Could you check a few things on this drawing? It's one solid part, dimensions in mm from its lowest x, y, z. A direction names the side the tool comes from. Give positions to 0.01 mm unless a question says otherwise; leave off trailing zeros. Order: outer loops, then holes, each group sorted by start corner. A loop starts at its lowest first (then second) coordinate and runs counter-clockwise, first axis right, second up.
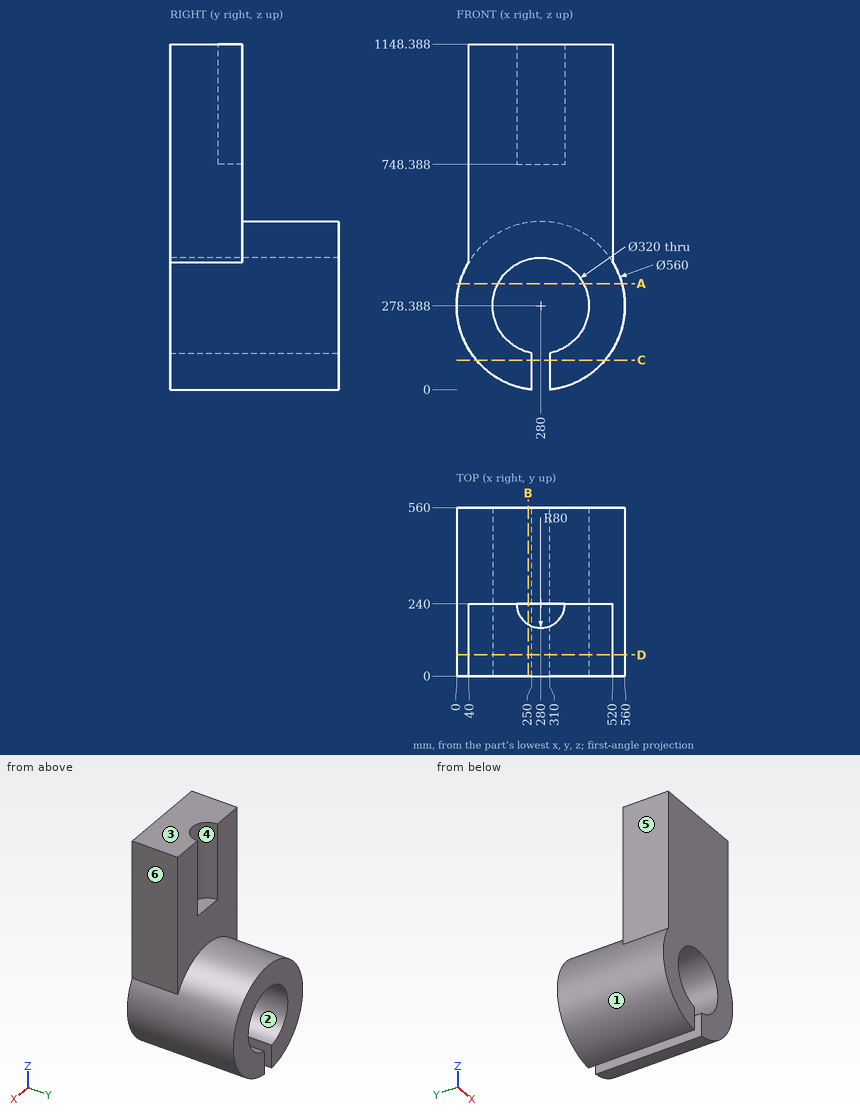
Q1. If we section it at D-D on y = 70.5: List the corners of the cut face in (x, z) for me, plus the area to 3 significant figures.
Filled sheet:
outline: (40, 422.61) arc R280 ccw to (250, 0) - (250, 121.23) arc R160 cw (long way) to (310, 121.23) - (310, 0) arc R280 ccw to (520, 422.61) - (520, 1148.39) - (40, 1148.39) - close
area: 461,000 mm2
Q2. I need wall thicknesses on L1, parallel to Y at x = 179.5, z = 619.5; L2, parallel to Z at x = 286.5, y = 80.5; L3, parallel to X at y = 77, z = 866.5. Which ranges of each line are inside material? Lowest first, please.
Filled sheet:
L1: y = 0 to 240
L2: z = 438.26 to 1148.39
L3: x = 40 to 520
Q3. If we section it at C-C on z = 98: List the corners of the cut face in (x, y) for me, plus the area to 3 significant figures.
Filled sheet:
outline: (65.85, 0) - (250, 0) - (250, 560) - (65.85, 560) - close; (310, 0) - (494.15, 0) - (494.15, 560) - (310, 560) - close
area: 206,000 mm2
Q4. If we section it at A-A on z = 352: List the corners of the cut face in (x, y) for me.
Filled sheet:
outline: (9.85, 0) - (137.94, 0) - (137.94, 560) - (9.85, 560) - close; (422.06, 0) - (550.15, 0) - (550.15, 560) - (422.06, 560) - close
Q5. I'm going to push flat-ended pins straight in: P1, Ø24, axis at x = 302, y = 180, coming from the +Z side; P2, Ø1, axis at x = 479, y = 241, coming from the +Z side; P3, Ø12, axis at x = 359.5, y = 499.5, coming from the -Z side. Where does each tip first touch, or does it pass through?
Filled sheet:
P1: stops at z = 748.39
P2: stops at z = 475.87
P3: stops at z = 8.21
Q6. If we section it at B-B on x = 238: List the corners of the cut face in (y, z) for me.
Filled sheet:
outline: (0, 1.56) - (560, 1.56) - (560, 124) - (0, 124) - close; (0, 432.78) - (560, 432.78) - (560, 555.22) - (240, 555.22) - (240, 748.39) - (171.91, 748.39) - (171.91, 1148.39) - (0, 1148.39) - close
Q7. For the marked faces 4, 5 and 6, which set-ups out of +Z, -Z, +X, -X, +Y, -Y let a thin tool reach every point of the face, with its end or its side?
Filled sheet:
face 4: +Z, +Y
face 5: +Z, -X, +Y, -Y
face 6: +Z, +X, +Y, -Y
Q8. Thinking about a two-plate mould opening in X: for the marked faces 1, 2 and 3, which applies, released by +X, released by -X, zero draft, split by the parting line, or undercut?
Filled sheet:
face 1: split by the parting line
face 2: undercut
face 3: zero draft
